Verification items for the finished model (mm, model axes). Face numbers are marked on the shaded views. A direction names the side the tool comes from. Coordinates: 2 decimals unless noted, no trailing zeros. Loops run counter-clockwise (first coordinate to the right, second up) from the corner with the lowest first, then second, coordinate; pieces in that order, holes last. Notation, with made-up numbers: (11, -39.5) - (23, -39.5) arc R24 cw to (23, -0.5) - close; hole circle Ø1 at (77.25, 67.25). An arc over 180 degrees is marked (long way). One line per item, written item: value. Start each with the question number.
(1) Section check B-B (y = 18.5). Record the boundary of the cut face in (x, z), plus the area to 3 significant figures.
(2) Thickness scan on probe 1 along Y at (x, z) = (1, 25.5) (3 decimals); probe 2 along Y at (x, z) = (-1.5, 11) (3 decimals); probe 3 along Z at (x, y) = (6.5, 36.5). Record the ranges inside material, lowest first. Write a range as [from, to].
(3) Set-up check for the marked faces 5 and 6: record each of +Z, -Z, +X, -X, +Y, -Y from which the full face is reachable in a straight line by a thin tool's end or side.
(4) Section check A-A (x = 0). Record the boundary of the cut face in (y, z) (3 decimals).
(5) Draft check along X on the marked faces 1, 2, 3 and 4. Enter one of: +X half, -X half, draft (parallel to the pull), parting line (faces both ways), or undercut.
(6) Section check D-D (x = 4.5). Record the boundary of the cut face in (y, z) (3 decimals), plus the area to 3 significant figures.
(7) Gauge pin test, flat ends, axial feed: P1, Ø4.5, axis at x = 0, z = 24.55, coming from the +Y side (3 decimals); P2, Ø11, axis at x = 0.5, z = 11.5, coming from the -Y side; P3, Ø4, axis at x = 9.5, y = 19.5, coming from the -Z side. Record the tip position at first contact, or that the pin passes through.
(8) Section check C-C (z = 0). Record the boundary of the cut face in (x, y), plus the area to 3 significant figures.
```python
from build123d import *

# Parameters (mm, degrees)
SKETCH_1_R           = 11
EXTRUDE_1_DEPTH      = 50
SKETCH_2_R           = 7.5
CUT_EXTRUDE_1_DEPTH  = 53.364109846
SKETCH_4_R           = 1.935
CUT_EXTRUDE_4_DEPTH  = 50
EXTRUDE_2_DEPTH      = 10
EXTRUDE_2_DEPTH_BACK = 10
SKETCH_11_W          = 22
SKETCH_11_H          = 22.065
SKETCH_35_W          = 2
SKETCH_35_H          = 4.895889032
CUT_EXTRUDE_5_DEPTH  = 19
SKETCH_36_R          = 2
CUT_EXTRUDE_6_DEPTH  = 19
SKETCH_38_W          = 35.522416841
SKETCH_38_H          = 17.874337136
CUT_EXTRUDE_7_DEPTH  = 29


with BuildPart() as part:
    # Sketch 1 → Extrude 1 (new body)
    with BuildSketch(Plane(origin=(0, 0, 0), x_dir=(1, 0, 0), z_dir=(0, 1, 0))):
        with Locations(Location((0, 0, 0), (0, 0, 270))):
            Circle(SKETCH_1_R)
    extrude(amount=EXTRUDE_1_DEPTH)

    # Sketch 2 → Cut-Extrude 1 (cut, through all)
    with BuildSketch(Plane(origin=(0, 50, 0), x_dir=(1, 0, 0), z_dir=(0, 1, 0))):
        with Locations(Location((0, 0, 0), (0, 0, 270))):
            Circle(SKETCH_2_R)
    extrude(amount=-CUT_EXTRUDE_1_DEPTH, mode=Mode.SUBTRACT)

    # Sketch 4 → Cut-Extrude 4 (cut)
    with BuildSketch(Plane.XY.offset(18)):
        with Locations((0, 40)):
            Circle(SKETCH_4_R)
    extrude(amount=-CUT_EXTRUDE_4_DEPTH, mode=Mode.SUBTRACT)

    # Sketch 11 → Extrude 2 (add, two sides: drawn at the far end of the back side and taken through both)
    with BuildSketch(Plane.XY.offset(18).offset(-EXTRUDE_2_DEPTH_BACK)):
        with Locations((0, 11.0325)):
            Rectangle(SKETCH_11_W, SKETCH_11_H)
    extrude(amount=EXTRUDE_2_DEPTH + EXTRUDE_2_DEPTH_BACK)

    # Sketch 35 → Cut-Extrude 5 (cut)
    with BuildSketch(Plane(origin=(0, 22.065, 0), x_dir=(1, 0, 0), z_dir=(0, 1, 0))):
        with Locations((0, -28)):
            Rectangle(SKETCH_35_W, SKETCH_35_H)
    extrude(amount=-CUT_EXTRUDE_5_DEPTH, mode=Mode.SUBTRACT)

    # Sketch 36 → Cut-Extrude 6 (cut)
    with BuildSketch(Plane(origin=(0, 22.065, 0), x_dir=(1, 0, 0), z_dir=(0, 1, 0))):
        with Locations((0, -24.552055484)):
            Circle(SKETCH_36_R)
    extrude(amount=-CUT_EXTRUDE_6_DEPTH, mode=Mode.SUBTRACT)

    # Sketch 38 → Cut-Extrude 7 (cut)
    with BuildSketch(Plane(origin=(11, 0, 0), x_dir=(0, 0, -1), z_dir=(1, 0, 0))):
        with Locations((-6.652230971, 8.407788312)):
            Rectangle(SKETCH_38_W, SKETCH_38_H)
    extrude(amount=-CUT_EXTRUDE_7_DEPTH, mode=Mode.SUBTRACT)


solid = part.part
```
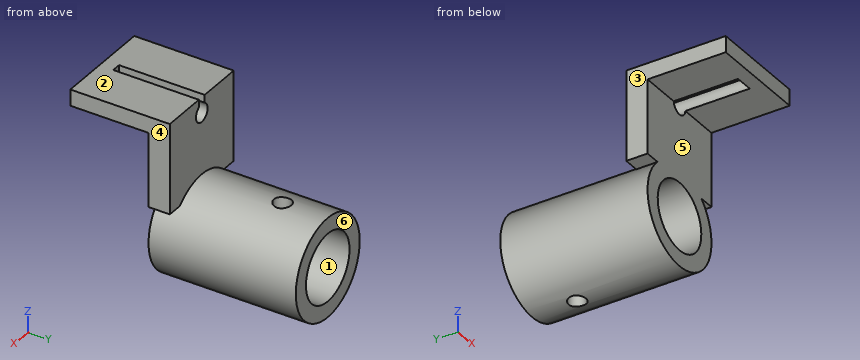
Responses:
1. outline: (-11, 8) - (-7.55, 8) arc R11 ccw (long way) to (7.55, 8) - (11, 8) - (11, 28) - (1, 28) - (1, 26.28) arc R2 cw (long way) to (-1, 26.28) - (-1, 28) - (-11, 28) - close; hole circle Ø15 at (0, 0)
1. area: 597 mm²
2. probe 1: y = [0, 3.065]
2. probe 2: y = [17.345, 22.065]
2. probe 3: z = [-8.87, -3.74], [3.74, 8.87]
3. face 5: -Z, +X, -X, -Y
3. face 6: +Z, -Z, +X, -X, +Y
4. outline: (0, 24.413) - (3.065, 24.413) - (3.065, 28) - (0, 28) - close; (17.345, -11) - (38.065, -11) - (38.065, -7.5) - (17.345, -7.5) - close; (17.345, 7.5) - (38.065, 7.5) - (38.065, 11) - (22.065, 11) - (22.065, 22.552) - (17.345, 22.552) - close; (41.935, -11) - (50, -11) - (50, -7.5) - (41.935, -7.5) - close; (41.935, 7.5) - (50, 7.5) - (50, 11) - (41.935, 11) - close
5. face 1: undercut
5. face 2: draft
5. face 3: -X half
5. face 4: +X half
6. outline: (0, 24.413) - (17.345, 24.413) - (17.345, 6) - (50, 6) - (50, 10.037) - (22.065, 10.037) - (22.065, 28) - (0, 28) - close; (17.345, -10.037) - (50, -10.037) - (50, -6) - (17.345, -6) - close
6. area: 411 mm²
7. P1: stops at y = 22.065
7. P2: stops at y = 17.34
7. P3: stops at z = -8.05
8. outline: (-11, 17.34) - (-7.5, 17.34) - (-7.5, 50) - (-11, 50) - close; (7.5, 17.34) - (11, 17.34) - (11, 50) - (7.5, 50) - close
8. area: 229 mm²
